Verification items for the finished model (mm, model axes). A direction names the side the tool comes from. Round coordinates to 2 decimals unless told otherwise and drop trailing zeros. Write each loop counter-clockwise with the first axis right and the second up, starting at its lowest first coordinate (ties: lowest second). Pieces come first, ordered by that corner, then holes. Notation, with made-up numbers: M -11,-9 L 44,-9 A27 ccw 44,26 Z; hole C -23.5,13 d6. An arc over 180 degrees is marked long. One line per item, written item: value. Start each with the question number.
Item 1: Section check B-B, the plane y = 86. Record the cut outline in (x, z).
Item 2: Gauge pin test, flat ends, axial feed: pin 1 (3 mm diameter, centred on x = -22, y = 150, fed in from +Z); pin 2 (12 mm diameter, centred on x = 101, y = 128.5, fed in from +Z); pin 3 (4.5 mm diameter, centred on x = -19.5, z = 133, fed in from -Y) (3 decimals). Record the tip position at first contact, or that the pin passes through.
Item 3: Section check C-C, the plane y = 24.5. Record the cut outline in (x, z), then the cut area to 3 significant figures.
Item 4: Section check D-D, the plane z = 0. Record the cut outline in (x, y), then the cut area to 3 significant figures.
Item 5: Tool access check on faces 1 (the face through (-42.862, 21, 134)), 2 (the face through (-1, 97, 139.2)), 3 (the face through (-2, 146.05, -11)). Record the directions out of +Z, -Z, +X, -X, +Y, -Y that give a thin tool (end or side, any length) a straight path to the whole face; none if there is none.
Item 6: Thickness scan on probe 1 along X at (y, z) = (72, 0); probe 2 along Z at (x, y) = (0, 141.5); probe 3 along X at (y, z) = (19.5, -6). Record the ranges inside material, lowest first. Write a range as from..to.
Item 7: Draft check along X on faces 4 (the face through (66.745, 75.133, 151.817)), 5 (the face through (-43.1, 0, 131.1)), 6 (the face through (-67.513, 75.133, 152.175)), 7 (the face through (6.969, 75.133, -189.872)). Enter one of: +X half, -X half, draft (parallel to the pull), parting line (faces both ways), or undercut.
Item 8: Section check A-A, the plane x = 0. Record the cut outline in (y, z), then the cut area to 3 significant figures.
from build123d import *

# Parameters (mm, degrees)
BOSS_EXTRUDE1_DEPTH     = 152.4
SHELL2_T                = -12.7
CUT_EXTRUDE1_DEPTH      = 43.175
CUT_EXTRUDE2_DEPTH      = 309.910601955
CUT_EXTRUDE2_DEPTH_BACK = 309.910601955
SKETCH3_W               = 90
SKETCH3_H               = 40
SKETCH4_W               = 13.97
SKETCH4_H               = 33.025
CUT_EXTRUDE3_DEPTH      = 12.7
SKETCH5_W               = 90
SKETCH5_H               = 40
CUT_EXTRUDE4_DEPTH      = 6.35


with BuildPart() as part:
    # Sketch1 → Boss-Extrude1 (new body)
    with BuildSketch(Plane(origin=(0, 0, 0), x_dir=(1, 0, 0), z_dir=(0, 1, 0))):
        with BuildLine():
            Line((-39.6875, -139.2), (39.6875, -139.2))
            Line((39.6875, -139.2), (94.570201191, -164.792223866))
            ThreePointArc((94.570201191, -164.792223866), (0, 190), (-94.570201191, -164.792223866))
            Line((-94.570201191, -164.792223866), (-39.6875, -139.2))
        make_face()
    extrude(amount=BOSS_EXTRUDE1_DEPTH)

    # Shell2
    shell2_openings = [part.faces().sort_by_distance(p)[0] for p in [
        (0, 0, -10.230254614),
    ]]
    offset(amount=SHELL2_T, openings=shell2_openings, kind=Kind.INTERSECTION)

    # Sketch2 → Cut-Extrude1 (cut)
    with BuildSketch(Plane.XZ):
        Polygon((-42.503022216, 126.5), (42.503022216, 126.5), (42.8625, 126.667627244), (42.8625, 140.680526815), (39.6875, 139.2), (-39.6875, 139.2), (-42.8625, 140.680526815), (-42.8625, 126.667627244), align=None)
    extrude(amount=-CUT_EXTRUDE1_DEPTH, mode=Mode.SUBTRACT)

    # Sketch3 → Cut-Extrude2 (cut, two sides: drawn at the far end of the back side and taken through both)
    with BuildSketch(Plane(origin=(0, 152.4, 0), x_dir=(1, 0, 0), z_dir=(0, 1, 0)).offset(-CUT_EXTRUDE2_DEPTH_BACK)):
        with Locations((0, -76.2)):
            Rectangle(SKETCH3_W, SKETCH3_H)
    extrude(amount=CUT_EXTRUDE2_DEPTH + CUT_EXTRUDE2_DEPTH_BACK, mode=Mode.SUBTRACT)

    # Sketch4 → Cut-Extrude3 (cut)
    with BuildSketch(Plane.XY.offset(139.2)):
        with Locations((0, 59.6875)):
            Rectangle(SKETCH4_W, SKETCH4_H)
    extrude(amount=-CUT_EXTRUDE3_DEPTH, mode=Mode.SUBTRACT)

    # Sketch5 → Cut-Extrude4 (cut)
    with BuildSketch(Plane.XZ.offset(-139.7)):
        with BuildLine():
            Line((42.503022216, 126.5), (-42.503022216, 126.5))
            Line((-42.503022216, 126.5), (-93.832389801, 150.435277193))
            ThreePointArc((-93.832389801, 150.435277193), (0, -177.3), (93.832389801, 150.435277193))
            Line((93.832389801, 150.435277193), (42.503022216, 126.5))
        make_face()
        with Locations((0, 76.2)):
            Rectangle(SKETCH5_W, SKETCH5_H, mode=Mode.SUBTRACT)
    extrude(amount=-CUT_EXTRUDE4_DEPTH, mode=Mode.SUBTRACT)


solid = part.part
Response values:
1. outline: M -94.57,164.79 A190 ccw long 94.57,164.79 L 39.69,139.2 L -39.69,139.2 Z; hole M -93.83,150.44 A177.3 ccw long 93.83,150.44 L 42.5,126.5 L -42.5,126.5 Z
2. pin 1: stops at z = 139.2
2. pin 2: stops at z = 164.54
2. pin 3: stops at y = 43.175
3. outline: M -94.57,164.79 A190 ccw long 94.57,164.79 L 42.86,140.68 L 42.86,126.67 L 93.83,150.44 A177.3 cw long -93.83,150.44 L -42.86,126.67 L -42.86,140.68 Z
3. area: 13,600 mm2
4. outline: M -190,0 L -177.3,0 L -177.3,146.05 L 177.3,146.05 L 177.3,0 L 190,0 L 190,152.4 L -190,152.4 Z
4. area: 6,120 mm2
5. face 1: +Z, -Y
5. face 2: +Z, +Y, -Y
5. face 3: -Y
6. probe 1: x = -190..-177.3, 177.3..190
6. probe 2: z = -190..-177.3, 126.5..139.2
6. probe 3: x = -189.91..-177.2, 177.2..189.91
7. face 4: undercut
7. face 5: draft
7. face 6: undercut
7. face 7: parting line
8. outline: M 0,-190 L 152.4,-190 L 152.4,56.2 L 146.05,56.2 L 146.05,-177.3 L 0,-177.3 Z; M 76.2,126.5 L 146.05,126.5 L 146.05,96.2 L 152.4,96.2 L 152.4,139.2 L 76.2,139.2 Z
8. area: 4,580 mm2
